```python
from build123d import *

# Parameters (mm, degrees)
SKETCH1_W           = 78
SKETCH1_H           = 80
BOSS_EXTRUDE1_DEPTH = 2
SKETCH2_W           = 34.450546123
SKETCH2_H           = 3.156291742
CUT_EXTRUDE1_DEPTH  = 10
SKETCH3_W           = 10.842335807
SKETCH3_H           = 80
BOSS_EXTRUDE2_DEPTH = 7.5
SKETCH4_R           = 2.5
CUT_EXTRUDE2_DEPTH  = 20
SKETCH5_R           = 5
CUT_EXTRUDE3_DEPTH  = 5
FILLET1_R           = 5
SKETCH8_W           = 49.971339188
SKETCH8_H           = 59.988397901
BOSS_EXTRUDE3_DEPTH = 3
FILLET3_R           = 3
SKETCH9_W           = 34.450546123
SKETCH9_H           = 3.156291742
CUT_EXTRUDE4_DEPTH  = 3
CUT_EXTRUDE4_DRAFT  = 27


# Some blends are built 0.0001 mm under size
with BuildPart() as part:
    # Sketch1 → Boss-Extrude1 (new body)
    with BuildSketch(Plane.XY):
        with Locations((-26.054678924, 10.907965965)):
            Rectangle(SKETCH1_W, SKETCH1_H)
    extrude(amount=BOSS_EXTRUDE1_DEPTH)

    # Sketch2 → Cut-Extrude1 (cut)
    with BuildSketch(Plane(origin=(0, 0, 0), x_dir=(-1, 0, 0), z_dir=(0, 0, -1))):
        with Locations((18.339951986, 15.829820094)):
            Rectangle(SKETCH2_W, SKETCH2_H)
    extrude(amount=-CUT_EXTRUDE1_DEPTH, mode=Mode.SUBTRACT)

    # Sketch3 → Boss-Extrude2 (add)
    with BuildSketch(Plane(origin=(0, 0, 0), x_dir=(-1, 0, 0), z_dir=(0, 0, -1))):
        with Locations((56.706233252, 10.907965965)):
            Rectangle(SKETCH3_W, SKETCH3_H)
    extrude(amount=BOSS_EXTRUDE2_DEPTH)

    # Sketch4 → Cut-Extrude2 (cut)
    with BuildSketch(Plane(origin=(0, 0, -7.5), x_dir=(-1, 0, 0), z_dir=(0, 0, -1))):
        with Locations((57.617298924, -1.683561388)):
            Circle(SKETCH4_R)
    extrude(amount=-CUT_EXTRUDE2_DEPTH, mode=Mode.SUBTRACT)

    # Sketch5 → Cut-Extrude3 (cut)
    with BuildSketch(Plane.XY.offset(2)):
        with Locations((-57.617298924, -1.683561388)):
            Circle(SKETCH5_R)
    extrude(amount=-CUT_EXTRUDE3_DEPTH, mode=Mode.SUBTRACT)

    # Fillet1
    # the kernel refuses this fillet: 5 mm, written as the material it adds along each edge
    with BuildSketch(Plane(origin=(-51.285065348, 50.907965965, 0), x_dir=(1, 0, 0), z_dir=(0, -1, 0))) as fillet1_piece_1:
        with BuildLine():
            CenterArc((FILLET1_R, -FILLET1_R), FILLET1_R, 90, 90)
            Line((0, -FILLET1_R), (0, 0))
            Line((0, 0), (FILLET1_R, 0))
        make_face()
    extrude(amount=80)
    # the kernel refuses this fillet: 5 mm, written as the material it adds along each edge
    with BuildSketch(Plane(origin=(-62.127401155, -29.092034035, 0), x_dir=(0, 0, -1), z_dir=(0, 1, 0))) as fillet1_2_piece_1_section:
        with BuildLine():
            CenterArc((4.550145333, 5), FILLET1_R, 204.490631369, 65.509368631)
            Line((0, 2.927277769), (0, 0))
            Line((0, 0), (4.550145333, 0))
        make_face()
    fillet1_2_piece_1 = extrude(amount=36.625369426, mode=Mode.PRIVATE)
    fillet1_2_piece_1 = split(fillet1_2_piece_1, bisect_by=Plane(origin=(-62.127401155, -29.092034035, -3), z_dir=(0, 0, -1)), keep=Keep.TOP, mode=Mode.PRIVATE)
    add(fillet1_2_piece_1)
    with BuildSketch(Plane(origin=(-62.127401155, -29.092034035, 0), x_dir=(0, 0, -1), z_dir=(0, 1, 0))) as fillet1_2_piece_2_section:
        with BuildLine():
            CenterArc((4.550145333, 5), FILLET1_R, 204.490631369, 65.509368631)
            Line((0, 2.927277769), (0, 0))
            Line((0, 0), (4.550145333, 0))
        make_face()
    fillet1_2_piece_2 = extrude(amount=36.625369426, mode=Mode.PRIVATE)
    fillet1_2_piece_2 = fillet1_2_piece_2 - Plane(origin=(-57.617298924, -1.683561388, 0), x_dir=(1, 0, 0), z_dir=(0, 0, 1)) * Cylinder(5, 92, mode=Mode.PRIVATE)
    add(fillet1_2_piece_2)
    # the kernel refuses this fillet: 5 mm, written as the material it adds along each edge
    with BuildSketch(Plane(origin=(-62.127401155, 7.533335391, 0), x_dir=(-1, 0, 0), z_dir=(0, 1, 0))) as fillet1_3_piece_1:
        with BuildLine():
            CenterArc((5, -4.550145333), FILLET1_R, 114.490631369, 65.509368631)
            Line((0, -4.550145333), (0, 0))
            Line((0, 0), (2.927277769, 0))
        make_face()
    extrude(amount=43.374630574)
    # the kernel refuses this fillet: 5 mm, written as the material it takes off along each edge

    # Sketch8 → Boss-Extrude3 (add)
    with BuildSketch(Plane.XY.offset(2)):
        with Locations((-17.086726302, 15.98380471)):
            Rectangle(SKETCH8_W, SKETCH8_H)
    extrude(amount=BOSS_EXTRUDE3_DEPTH)

    # Fillet3
    fillet3_edges = [part.edges().sort_by_distance(p)[0] for p in [
        (-17.086726302, -14.010394241, 5),
        (-17.086726302, 45.97800366, 5),
    ]]
    fillet(fillet3_edges, radius=FILLET3_R - 0.0001)  # a hair under: the kernel refuses the full size


with BuildPart() as cut_extrude4_tool:
    # Sketch9 → Cut-Extrude4 (with draft: the straight prism first)
    with BuildSketch(Plane(origin=(0, 0, 2), x_dir=(-1, 0, 0), z_dir=(0, 0, -1))):
        with Locations((18.339951986, 15.829820094)):
            Rectangle(SKETCH9_W, SKETCH9_H)
    extrude(amount=-CUT_EXTRUDE4_DEPTH)
    # Cut-Extrude4: the draft: its side faces are tilted about the plane it starts from
    cut_extrude4_sides = [cut_extrude4_tool.faces().sort_by_distance(p)[0] for p in [
        (-18.339951986, 17.407965965, 3.5),
        (-1.114678924, 15.829820094, 3.5),
        (-18.339951986, 14.251674223, 3.5),
        (-35.565225047, 15.829820094, 3.5),
    ]]
    draft(cut_extrude4_sides, Plane(origin=(0, 0, 2), x_dir=(-1, 0, 0), z_dir=(0, 0, -1)), CUT_EXTRUDE4_DRAFT)


with BuildPart() as part_1:
    add(part.part)

    # Cut-Extrude4: cut by cut_extrude4_tool
    add(cut_extrude4_tool.part, mode=Mode.SUBTRACT)


solid = part_1.part
```
Part model, mm, in its own coordinate system. A direction names the side the tool comes from. Round coordinates to 2 decimals unless told otherwise and drop trailing zeros. Loops run counter-clockwise (first coordinate to the right, second up) from the corner with the lowest first, then second, coordinate; pieces in that order, holes last. Notation, with made-up numbers: (-36.5, 21.5) -> (-10.5, 21.5) arc R24 ccw to (-10.5, 46.5) -> close; hole circle Ø10 at (21, 50). An arc over 180 degrees is marked (long way). Use CSV: the item, a comma, the result in double quotes. Start each with the question number.
1) Cut at B-B, the plane z = 4. Write the cut outline in (x, y), plus the area to 3 significant figures.
2) Cut at D-D, the plane y = 26. Write the cut outline in (x, z), plus the area to 3 significant figures.
3) Which spindle directions (+Z, -Z, +X, -X, +Y, -Y) get a long thin tool onto all of the face, cutting with end or side? Do faces 5 (the flat face through (7.899, 16, 3)), 6 (the flat face through (-0.191, 15.786, 3.812)), 7 (the flat face through (-18, 14.252, 1)). Say none if no direction does.
4) Pull direction X, two halves, no side cores. Call faces 1 (the flat face through (-17, 11, 0)), 2 (the flat face through (-56, -4, -3)), 3 (the flat face through (-62.127, 10, -6)), 4 (the flat face through (-18.08, 18.16, 3.48)): +X half, -X half, draft (parallel to the pull), parting line (faces both ways), or undercut.
5) Drop flat-ended pins along their axis: P1, Ø2, axis at x = -33, y = -10.5, coming from the -Z side; P2, Ø0.9, axis at y = 30.5, z = 3, coming from the -X side; P3, Ø1.2, axis at y = 16.5, z = -6.5, coming from the +X side; P4, Ø6.5, axis at x = -57.62, y = -1.68, coming from the -Z side. Give the stop position or say it passes through.
6) Wall check: L1, parallel to X at y = -2, z = -6.5; L2, parallel to Z at x = 4.5, y = -7.5; L3, parallel to X at y = -4, z = 2.25. Give the ranges that are in metal, low to high. Write a range as [from, to].
Determined:
1,outline,"(-42.07, -13.25) -> (7.9, -13.25) -> (7.9, 45.21) -> (-42.07, 45.21) -> close; hole (-36.58, 13.23) -> (-0.1, 13.23) -> (-0.1, 18.43) -> (-36.58, 18.43) -> close"
1,area,"2,730 mm2"
2,outline,"(-65.05, 0) arc R5 cw to (-62.13, -4.55) -> (-62.13, -7.5) -> (-51.29, -7.5) -> (-51.29, -5) arc R5 cw to (-46.29, 0) -> (12.95, 0) -> (12.95, 2) -> (7.9, 2) -> (7.9, 5) -> (-42.07, 5) -> (-42.07, 2) -> (-65.05, 2) -> close"
2,area,"396 mm2"
3,face 5,"+Z, +X, +Y, -Y"
3,face 6,"+Z"
3,face 7,"+Z, -Z"
4,face 1,"draft"
4,face 2,"undercut"
4,face 3,"-X half"
4,face 4,"undercut"
5,P1,"stops at z = 0"
5,P2,"stops at x = -42.07"
5,P3,"stops at x = -51.29"
5,P4,"stops at z = -7.5"
6,L1,"x = [-62.13, -60.1], [-55.14, -51.29]"
6,L2,"z = [0, 5]"
6,L3,"x = [-42.07, 7.9]"
